```python
from build123d import *

# Parameters (mm, degrees)
SKETCH_R       = 1.75
PAD_DEPTH      = 8
THICKNESS001_T = 1
SKETCH013_W    = 12.495425
SKETCH013_H    = 4.952306
POCKET_DEPTH   = 6.751


with BuildPart() as part:
    # Sketch → Pad (new body)
    with BuildSketch(Plane.XY):
        Circle(SKETCH_R)
    extrude(amount=PAD_DEPTH)

    # Thickness001
    thickness001_openings = [part.faces().sort_by_distance(p)[0] for p in [
        (0, 0, 8),
    ]]
    offset(amount=THICKNESS001_T, openings=thickness001_openings, kind=Kind.INTERSECTION)

    # Sketch013 → Pocket (cut, through all)
    with BuildSketch(Plane.YZ.offset(4)):
        with Locations((0.810456, -2.476153)):
            Rectangle(SKETCH013_W, SKETCH013_H)
    extrude(amount=-POCKET_DEPTH, mode=Mode.SUBTRACT)


solid = part.part
```
CAD build for the part. Positions are in the model's coordinates, mm. Round coordinates to 2 decimals unless told otherwise and drop trailing zeros. Order: outer loops, then holes, each group sorted by start corner. A loop starts at its lowest first (then second) coordinate and runs counter-clockwise, first axis right, second up. Notation, with made-up numbers: (-2, 6) -> (55, 6) arc R19 ccw to (55, 20) -> close; hole circle Ø6 at (-35.75, 61.25). An arc over 180 degrees is marked (long way). Write item = value, one per line.
(1) Drill centre lines: L1, parallel to Y at x = 0, z = 6; L2, parallel to Y at x = -1.4, z = 6; L3, parallel to X at y = 1, z = 2.5. Where is each one in solid material? Low to high.
Answers follow:
L1 = -2.75 to -1.75, 1.75 to 2.75
L2 = -2.37 to -1.05, 1.05 to 2.37
L3 = -2.56 to -1.44, 1.44 to 2.56
(2) Cut at C-C (z = 4.25). Write the cut outline in (x, y), plus the area to 3 significant figures.
Answers follow:
outline = circle Ø5.5 at (0, 0); hole circle Ø3.5 at (0, 0)
area = 14.1 mm²
(3) Cut at A-A (y = 0). Write the cut outline in (x, z).
Answers follow:
outline = (-2.75, 0) -> (-1.75, 0) -> (-1.75, 8) -> (-2.75, 8) -> close; (1.75, 0) -> (2.75, 0) -> (2.75, 8) -> (1.75, 8) -> close
(4) Cut at D-D (y = -2.4). Write the cut outline in (x, z), plus the area to 3 significant figures.
Answers follow:
outline = (-1.34, 0) -> (1.34, 0) -> (1.34, 8) -> (-1.34, 8) -> close
area = 21.5 mm²
(5) Flat gauge pins, fed straight in: P1, Ø1.5, axis at x = 1, z = 3, coming from the -Y side; P2, Ø1, axis at y = 2, z = 7, coming from the +X side; P3, Ø1.5, axis at x = 1, z = 3, coming from the +Y side. Where does each tip first touch, or does it go through?
Answers follow:
P1 = -2.74
P2 = 2.3
P3 = 2.74
(6) Pull direction X, two halves, no side cores. Call faces 1 (the cylindrical face through (-0.596, -2.685, 3.944)), 2 (the flat face through (-2, 0, 0)), 3 (the cylindrical face through (1.617, -0.67, 3.944)): +X half, -X half, draft (parallel to the pull), parting line (faces both ways), or undercut.
Answers follow:
face_1 = parting line
face_2 = draft
face_3 = undercut
